```python
from build123d import *

# Parameters (mm, degrees)
IZIM1_W                     = 20
IZIM1_H                     = 20
Y_KSEKLIK_EKSTR_ZYON1_DEPTH = 20
KES_EKSTR_ZYON1_DEPTH       = 20
IZIM3_W                     = 17.224679165
IZIM3_H                     = 17.248412117
KES_EKSTR_ZYON2_DEPTH       = 20
IZIM4_R                     = 2
KES_EKSTR_ZYON3_DEPTH       = 20
IZIM10_R                    = 2
KES_EKSTR_ZYON10_DEPTH      = 10


with BuildPart() as part:
    # Çizim1 → Yükseklik-Ekstrüzyon1 (new body)
    with BuildSketch(Plane.XY):
        with Locations((-13.172756411, -5.622082974)):
            Rectangle(IZIM1_W, IZIM1_H)
    extrude(amount=Y_KSEKLIK_EKSTR_ZYON1_DEPTH)

    # Çizim2 → Kes-Ekstrüzyon1 (cut)
    with BuildSketch(Plane.XY.offset(20)):
        Polygon((-3.172756411, 4.377917026), (-23.172756411, -15.622082974), (-23.172756411, 4.377917026), align=None)
    extrude(amount=-KES_EKSTR_ZYON1_DEPTH, mode=Mode.SUBTRACT)

    # Çizim3 → Kes-Ekstrüzyon2 (cut)
    with BuildSketch(Plane.XY.offset(20)):
        with Locations((-15.601705124, -3.767784851)):
            Rectangle(IZIM3_W, IZIM3_H)
    extrude(amount=-KES_EKSTR_ZYON2_DEPTH, mode=Mode.SUBTRACT)

    # Çizim4 → Kes-Ekstrüzyon3 (cut)
    with BuildSketch(Plane.ZY.offset(6.989365541)):
        with Locations((10, -4.007036941)):
            Circle(IZIM4_R)
    extrude(amount=-KES_EKSTR_ZYON3_DEPTH, mode=Mode.SUBTRACT)

    # Çizim10 → Kes-Ekstrüzyon10 (cut)
    with BuildSketch(Plane(origin=(0, -12.391990909, 0), x_dir=(1, 0, 0), z_dir=(0, 1, 0))):
        with Locations((-15.081060976, -10)):
            Circle(IZIM10_R)
    extrude(amount=-KES_EKSTR_ZYON10_DEPTH, mode=Mode.SUBTRACT)


solid = part.part
```
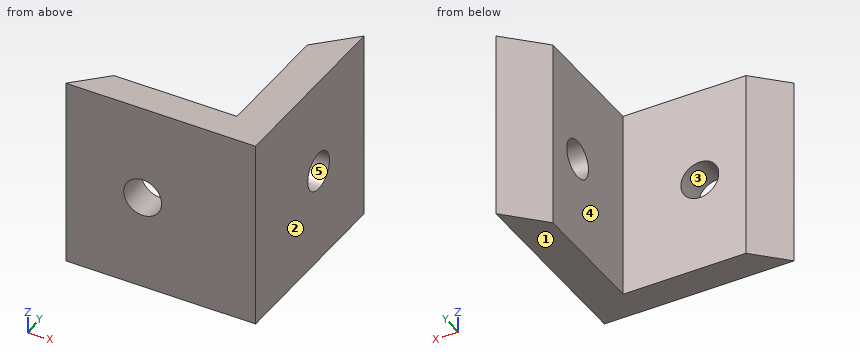
CAD build for the part. Positions are in the model's coordinates, mm. Face numbers are marked on the shaded views. A direction names the side the tool comes from. Coordinates: 2 decimals unless noted, no trailing zeros. Order: outer loops, then holes, each group sorted by start corner. A loop starts at its lowest first (then second) coordinate and runs counter-clockwise, first axis right, second up. Notation, with made-up numbers: M 67.5,-37 L 100.5,-37 A29 ccw 100.5,-4 Z; hole C 55.5,66.25 d5. An arc over 180 degrees is marked long. Answer as CSV lines item,"result".
1) 3-axis set-ups, long thin cutter, end or side, ignore diameter. For the marked faces 4 and 5: which of +Z, -Z, +X, -X, +Y, -Y reach the whole face in a straight line?
Verdict:
face 4,"+Z, -Z, -X, +Y"
face 5,"+X, -X"
2) Flat gauge pins, fed straight in: P1, Ø1, axis at y = -4, z = 12, coming from the -X side; P2, Ø10.5, axis at x = -12, z = 11, coming from the +Y side; P3, Ø5, axis at x = -10.5, y = -4.5, coming from the -Z side; P4, Ø3, axis at x = -14.5, z = 3, coming from the +Y side. Where does each tip first touch, or does it go through?
Verdict:
P1,"x = -6.99"
P2,"y = 0.8"
P3,"through"
P4,"y = -12.39"
3) Cut at A-A (z = 10). List the corners of the cut face in (x, y).
Verdict:
outline,"M -23.17,-15.62 L -17.08,-15.62 L -17.08,-12.39 L -19.94,-12.39 Z; M -13.08,-15.62 L -3.17,-15.62 L -3.17,-6.01 L -6.99,-6.01 L -6.99,-12.39 L -13.08,-12.39 Z; M -6.99,-2.01 L -3.17,-2.01 L -3.17,4.38 L -6.99,0.56 Z"
4) Cut at B-B (y = -3). List the corners of the cut face in (x, z), then the cut area to 3 significant figures.
Verdict:
outline,"M -6.99,0 L -3.17,0 L -3.17,8.27 L -6.99,8.27 Z; M -6.99,11.73 L -3.17,11.73 L -3.17,20 L -6.99,20 Z"
area,"63.1 mm2"
5) Cut at D-D (z = 15). List the corners of the cut face in (x, y).
Verdict:
outline,"M -23.17,-15.62 L -3.17,-15.62 L -3.17,4.38 L -6.99,0.56 L -6.99,-12.39 L -19.94,-12.39 Z"
6) Mould opens along Z. For the marked faces 1, 2 and 3 say: released by +Z, released by -Z, zero draft, split by the parting line, or undercut.
Verdict:
face 1,"released by -Z"
face 2,"zero draft"
face 3,"undercut"
7) Drill centre lines: L1, parallel to X at y = -11.75, z = 17; L2, parallel to Y at x = -15.5, z = 16.75; L3, parallel to X at y = -13.15, z = 10. Where is each one in solid material? Low to high. Write a range as from..to.
Verdict:
L1,"-6.99..-3.17"
L2,"-15.62..-12.39"
L3,"-20.7..-17.08, -13.08..-3.17"
8) Cut at C-C (x = -7.5). List the corners of the cut face in (y, z), then the cut area to 3 significant figures.
Verdict:
outline,"M -15.62,0 L -12.39,0 L -12.39,20 L -15.62,20 Z"
area,"64.6 mm2"
